from build123d import *

# Parameters (mm, degrees)
SKETCH_1_W          = 75
SKETCH_1_H          = 10
EXTRUDE_1_DEPTH     = 2
FILLET_1_R          = 5
SKETCH_3_R          = 2
CUT_EXTRUDE_1_DEPTH = 2


with BuildPart() as part:
    # 草图1 → 凸台-拉伸1 (new body)
    with BuildSketch(Plane.XY):
        Rectangle(SKETCH_1_W, SKETCH_1_H)
    extrude(amount=EXTRUDE_1_DEPTH)

    # 圆角1
    fillet_1_edges = [part.edges().sort_by_distance(p)[0] for p in [
        (37.5, -5, 1),
        (-37.5, -5, 1),
        (-37.5, 5, 1),
        (37.5, 5, 1),
    ]]
    fillet(fillet_1_edges, radius=FILLET_1_R - 0.0001)  # a hair under: the kernel refuses the full size

    # 草图3 → 切除-拉伸1 (cut)
    with BuildSketch(Plane.XY.offset(2)):
        with Locations((-32.5, 0)):
            Circle(SKETCH_3_R)
        with Locations(Location((32.5, 0, 0), (0, 0, 180))):
            Circle(SKETCH_3_R)
        Circle(SKETCH_3_R)
    extrude(amount=-CUT_EXTRUDE_1_DEPTH, mode=Mode.SUBTRACT)


solid = part.part
Build history of the part. All positions in model axes, mm. Coordinates: 2 decimals unless noted, no trailing zeros. Order: outer loops, then holes, each group sorted by start corner. A loop starts at its lowest first (then second) coordinate and runs counter-clockwise, first axis right, second up. Notation, with made-up numbers: (-13.5, 52) -> (39.5, 52) arc R22 cw to (39.5, 90) -> close; hole circle Ø4 at (60, 1.5). An arc over 180 degrees is marked (long way). One line per item, written item: value.
(1) Slice it at B-B, the plane z = 0.8. Count the separate pieces of the cut face and the enclosed holes in it, plus the area to 3 significant figures.
Checked values:
separate pieces: 1
enclosed holes: 3
area: 691 mm2
(2) Slice it at D-D, the plane y = -3.5. List the corners of the cut face in (x, z).
Checked values:
outline: (-36.07, 0) -> (36.07, 0) -> (36.07, 2) -> (-36.07, 2) -> close
(3) Slice it at C-C, the plane y = 3. List the corners of the cut face in (x, z).
Checked values:
outline: (-36.5, 0) -> (36.5, 0) -> (36.5, 2) -> (-36.5, 2) -> close
(4) Probe line 1 (X direction, y = -1, z = 0.9); line 2 (Y direction, x = -32.5, z = 0.75); line 3 (X direction, y = 1.5, z = 0.3). List the from-to ranges inside material, lowest first. Write a range as [from, to].
Checked values:
line 1: [-37.4, -34.23], [-30.77, -1.73], [1.73, 30.77], [34.23, 37.4]
line 2: [-5, -2], [2, 5]
line 3: [-37.27, -33.82], [-31.18, -1.32], [1.32, 31.18], [33.82, 37.27]
(5) Mould opens along X. For faces 1 (the cylindrical face through (30.592, -0.601, 1.014)), 2 (the cylindrical face through (0, -2, 1)), 3 (the cylindrical face through (-36.07, -3.5, 1.01)), 4 (the cylindrical face through (36, -3.57, 1.01)) say: pulls with the +X half, pulls with the -X half, needs draft (parallel to the pull), parting line crosses it, or undercut.
Checked values:
face 1: undercut
face 2: undercut
face 3: pulls with the -X half
face 4: pulls with the +X half
(6) Drop a flat-ended pin along its axis: pin 1 Ø2.5 at (x, y) = (-32.5, 0) entering from +Z. Give the stop position or say it passes through.
Checked values:
pin 1: through
(7) Slice it at A-A, the plane x = 0. List the corners of the cut face in (y, z).
Checked values:
outline: (-5, 0) -> (-2, 0) -> (-2, 2) -> (-5, 2) -> close; (2, 0) -> (5, 0) -> (5, 2) -> (2, 2) -> close
